```python
from build123d import *

# Parameters (mm, degrees)
SKETCH_1_R      = 1.7859375
SKETCH_1_R_2    = 1.5875
EXTRUDE_1_DEPTH = 1.5875


with BuildPart() as part:
    # 스케치1 → 보스-돌출1 (new body)
    with BuildSketch(Plane.XY):
        Polygon((0, 0), (203.2, 0), (203.2, 152.4), (-99.776362049, 233.582271537), (-175.976362049, 101.6), align=None)
        with Locations((2.041772846, 7.62)):
            Circle(SKETCH_1_R, mode=Mode.SUBTRACT)
        with Locations((177.8, 132.909894505)):
            Circle(SKETCH_1_R, mode=Mode.SUBTRACT)
        with Locations((190.5, 12.7)):
            Circle(SKETCH_1_R_2, mode=Mode.SUBTRACT)
        with Locations((101.6, 12.7)):
            Circle(SKETCH_1_R_2, mode=Mode.SUBTRACT)
        with Locations((25.4, 12.7)):
            Circle(SKETCH_1_R_2, mode=Mode.SUBTRACT)
        with Locations((-147.629316793, 99.898522628)):
            Circle(SKETCH_1_R_2, mode=Mode.SUBTRACT)
        with Locations((-81.638181024, 61.798522628)):
            Circle(SKETCH_1_R_2, mode=Mode.SUBTRACT)
        with Locations((-15.647045256, 23.698522628)):
            Circle(SKETCH_1_R_2, mode=Mode.SUBTRACT)
        with Locations((-95.127839421, 216.233748909)):
            Circle(SKETCH_1_R_2, mode=Mode.SUBTRACT)
        with Locations((-126.877839421, 161.241135768)):
            Circle(SKETCH_1_R_2, mode=Mode.SUBTRACT)
        Polygon((-106.301504082, 90.702595672), (-21.311447622, 41.633563696), (39.27303688, 25.4), (137.411100831, 25.4), align=None, mode=Mode.SUBTRACT)
        Polygon((177.8, 27.725834576), (177.8, 54.021849558), (-126.968392014, 135.684294077), (-140.116399505, 112.911277084), align=None, mode=Mode.SUBTRACT)
        with BuildLine():
            Line((-100.672377031, 181.230328063), (171.225996254, 108.375378518))
            ThreePointArc((171.225996254, 108.375378518), (155.802954744, 120.209894505), (153.265484012, 139.483898251))
            Line((153.265484012, 139.483898251), (-87.52436954, 204.003345056))
            Line((-87.52436954, 204.003345056), (-100.672377031, 181.230328063))
        make_face(mode=Mode.SUBTRACT)
        Polygon((-107.246380777, 169.843819566), (177.8, 93.465872032), (177.8, 67.169857049), (-120.394388268, 147.070802573), align=None, mode=Mode.SUBTRACT)
    extrude(amount=EXTRUDE_1_DEPTH)


solid = part.part
```
CAD build for the part. Positions are in the model's coordinates, mm. A direction names the side the tool comes from. Give positions to 0.01 mm unless a question says otherwise; leave off trailing zeros. Write each loop counter-clockwise with the first axis right and the second up, starting at its lowest first coordinate (ties: lowest second). Pieces come first, ordered by that corner, then holes. Notation, with made-up numbers: M -2.75,-23 L 39.25,-23 A17 ccw 39.25,-14 Z; hole C 26,-29 d6. An arc over 180 degrees is marked long. Return JSON: item names as keys, results as strings. Group by question number.
(1) Band-saw the part on C-C (z = 0.4). State how many separate pieces and enclosed holes the cut face has, and give its area (3 significant figures).
(2) Flat gauge pin, fed straight in: pin 1 Ø2.5 at (x, y) = (25.4, 12.7) entering from +Z. Where does the tip first touch, or does it go through?
(3) Mould opens along X. For faces 1 (the face through (53.833, 192.423, 0.783)), 2 (the face through (30.79, 106.56, 0.78)), 3 (the face through (-137.34, 168.52, 0.78)) say: pulls with the +X half, pulls with the -X half, needs draft (parallel to the pull), parting line crosses it, or undercut.
(4) Band-saw the part on D-D (x = -44). Give the cut face in (y, z).
(5) 3-axis set-ups, long thin cutter, end or side, ignore diameter. For faces 4 (the face through (33.28, 132.19, 0.78)), 5 (the face through (53, 92, 0)): which of +Z, -Z, +X, -X, +Y, -Y reach the whole face in a straight line?
(6) Drill centre lines: L1, parallel to Y at x = 64, z = 1.3; L2, parallel to Y at x = 0, z = 0.4; L3, parallel to Y at x = 154.5, z = 1.25. Where is each one in solid material? Low to high. Write a range as [from, to].
(7) Band-saw the part on B-B (x = 69). Give the cut face in (y, z).
(8) Band-saw the part on A-A (y = 173.5). Give the cut face in (x, z).
Entries:
{
 "1": {"separate pieces": "1", "enclosed holes": "14", "area": "35,800 mm^2"},
 "2": {"pin 1": "passes through"},
 "3": {"face 1": "pulls with the +X half", "face 2": "undercut", "face 3": "pulls with the -X half"},
 "4": {"outline": "M 25.4,0 L 54.73,0 L 54.73,1.59 L 25.4,1.59 Z; M 74.01,0 L 87.16,0 L 87.16,1.59 L 74.01,1.59 Z; M 113.45,0 L 126.6,0 L 126.6,1.59 L 113.45,1.59 Z; M 152.9,0 L 166.05,0 L 166.05,1.59 L 152.9,1.59 Z; M 192.34,0 L 218.64,0 L 218.64,1.59 L 192.34,1.59 Z"},
 "5": {"face 4": "+Z, -Z", "face 5": "-Z, +X, -X, +Y, -Y"},
 "6": {"L1": "y = [0, 25.4], [45.07, 58.22], [84.51, 97.66], [123.96, 137.11], [163.4, 189.7]", "L2": "y = [0, 35.92], [62.22, 75.37], [101.66, 114.81], [141.11, 154.26], [180.55, 206.85]", "L3": "y = [0, 33.97], [60.27, 73.41], [99.71, 112.86], [122.8, 165.45]"},
 "7": {"outline": "M 0,0 L 25.4,0 L 25.4,1.59 L 0,1.59 Z; M 43.73,0 L 56.88,0 L 56.88,1.59 L 43.73,1.59 Z; M 83.17,0 L 96.32,0 L 96.32,1.59 L 83.17,1.59 Z; M 122.62,0 L 135.77,0 L 135.77,1.59 L 122.62,1.59 Z; M 162.06,0 L 188.36,0 L 188.36,1.59 L 162.06,1.59 Z"},
 "8": {"outline": "M -134.46,0 L -71.82,0 L -71.82,1.59 L -134.46,1.59 Z; M 26.32,0 L 124.45,0 L 124.45,1.59 L 26.32,1.59 Z"}
}
